Geometry: final body of the model. Coordinates: model frame, mm. Face numbers are marked on the shaded views. Give positions to 0.01 mm unless a question says otherwise; leave off trailing zeros. Write each loop counter-clockwise with the first axis right and the second up, starting at its lowest first coordinate (ties: lowest second). Pieces come first, ordered by that corner, then holes. Notation, with made-up numbers: M 74.5,13.5 L 120.5,13.5 A12 cw 120.5,30.5 Z; hole C 72,63 d11. An arc over 180 degrees is marked long. Answer as a JSON object with one key per item and string values.
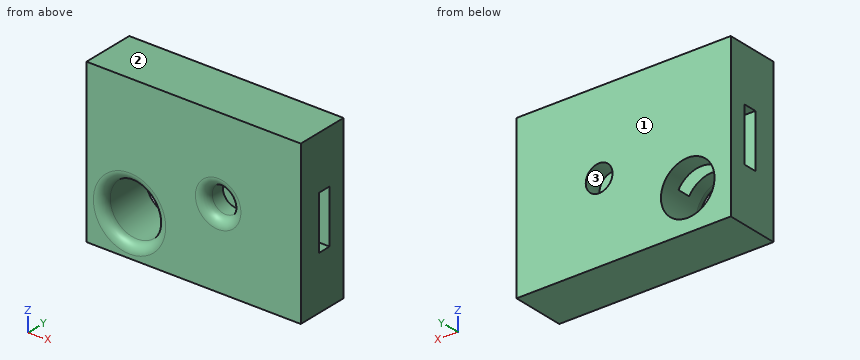
from build123d import *

# Parameters (mm, degrees)
F0_W     = 101.6
F0_H     = 76.2
F0_R     = 12.7
F0_R_2   = 6.35
F1_DEPTH = 25.4
F2_R     = 4.445
F3_W     = 6.35
F3_H     = 25.4
F4_DEPTH = 101.601


with BuildPart() as f1:
    # F0 (on Front) → F1 (new body)
    with BuildSketch(Plane.XZ):
        with Locations((4.996498, 19.05)):
            Rectangle(F0_W, F0_H)
        with Locations((-25.4, 0)):
            Circle(F0_R, mode=Mode.SUBTRACT)
        with Locations((16.619995, 18.330872)):
            Circle(F0_R_2, mode=Mode.SUBTRACT)
    extrude(amount=F1_DEPTH)

    # F2
    f2_edges = [f1.edges().sort_by_distance(p)[0] for p in [
        (-38.1, -25.4, 0),
        (10.269995, -25.4, 18.330872),
    ]]
    fillet(f2_edges, radius=F2_R)

    # F3 (on face) → F4 (cut, through all)
    with BuildSketch(Plane.YZ.offset(55.796498)):
        with Locations((-11.432072, 19.05)):
            Rectangle(F3_W, F3_H)
    extrude(amount=-F4_DEPTH, mode=Mode.SUBTRACT)


solid = f1.part
1) Cut plane D-D on x = -25.4. Return loops of the section in (y, z) (3 decimals), and give its area (3 significant figures).
Geometry check:
{"outline": "M -25.4,-19.05 L 0,-19.05 L 0,-12.7 L -20.955,-12.7 A4.445 ccw -25.4,-17.145 Z; M -25.4,17.145 A4.445 ccw -20.955,12.7 L -14.607,12.7 L -14.607,31.75 L -8.257,31.75 L -8.257,12.7 L 0,12.7 L 0,57.15 L -25.4,57.15 Z", "area": "1,160 mm2"}
2) Cut plane B-B on x = 3. Return loops of the section in (y, z).
Geometry check:
{"outline": "M -25.4,-19.05 L 0,-19.05 L 0,57.15 L -25.4,57.15 Z; hole M -14.61,6.35 L -8.26,6.35 L -8.26,31.75 L -14.61,31.75 Z"}
3) Cut plane A-A on y = -11.5. Return loops of the section in (x, z), and give its area (3 significant figures).
Geometry check:
{"outline": "M -45.8,-19.05 L 55.8,-19.05 L 55.8,6.35 L -14.4,6.35 A12.7 cw long -36.4,6.35 L -45.8,6.35 Z; M -45.8,31.75 L 55.8,31.75 L 55.8,57.15 L -45.8,57.15 Z", "area": "4,750 mm2"}
4) Pull-direction query (Z, two-part tool) for the marked faces 1, 2 and 3; classes: pulls with the +Z half, pulls with the -Z half, needs draft (parallel to the pull), parting line crosses it, or undercut.
Geometry check:
{"face 1": "needs draft", "face 2": "pulls with the +Z half", "face 3": "undercut"}
5) Line query: line 1 (Z direction, x = 15, y = -12.25); line 2 (Z direction, x = -25.4, y = -4.5); line 3 (Y direction, x = 35, z = 7). Output: solid intervals per line, ascending. Write a range as from..to.
Geometry check:
{"line 1": "z = -19.05..6.35, 31.75..57.15", "line 2": "z = -19.05..-12.7, 12.7..57.15", "line 3": "y = -25.4..-14.61, -8.26..0"}
6) Cut plane C-C on z = 0. Return loops of the section in (x, y) (1 decimal).
Geometry check:
{"outline": "M -45.8,-25.4 L -42.5,-25.4 A4.4 ccw -38.1,-21 L -38.1,0 L -45.8,0 Z; M -12.7,-21 A4.4 ccw -8.3,-25.4 L 55.8,-25.4 L 55.8,0 L -12.7,0 Z"}
